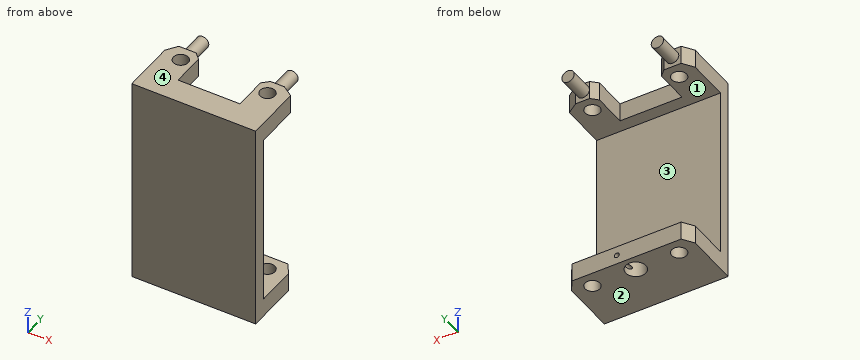
from build123d import *
from OCP.BRepFilletAPI import BRepFilletAPI_MakeChamfer

# Parameters (mm, degrees)
SKETCH1_W                      = 100
SKETCH1_H                      = 52
BOSS_EXTRUDE1_DEPTH            = 15
SKETCH2_R                      = 6
BOSS_EXTRUDE2_DEPTH            = 140
SKETCH3_W                      = 100
SKETCH3_H                      = 46
BOSS_EXTRUDE3_DEPTH            = 15
SKETCH4_W                      = 100
SKETCH4_H                      = 15
BOSS_EXTRUDE4_DEPTH            = 6
SKETCH5_W                      = 100
SKETCH5_H                      = 10
BOSS_EXTRUDE5_DEPTH            = 30
SKETCH6_W                      = 100
SKETCH6_H                      = 10
BOSS_EXTRUDE6_DEPTH            = 30
SKETCH7_W                      = 50
SKETCH7_H                      = 32
CUT_EXTRUDE1_DEPTH             = 168.705098312
SKETCH8_W                      = 6
SKETCH8_H                      = 1
SKETCH9_W                      = 6
SKETCH9_H                      = 1
SKETCH10_W                     = 6
SKETCH10_H                     = 1
SKETCH11_W                     = 6
SKETCH11_H                     = 1
SKETCH12_W                     = 6
SKETCH12_H                     = 140
F_10_0_10_DIAMETER_HOLE1_D     = 10
F_10_0_10_DIAMETER_HOLE1_DEPTH = 10
F_4_0_4_DIAMETER_HOLE1_D       = 4
F_4_0_4_DIAMETER_HOLE1_DEPTH   = 20
F_16_0_16_DIAMETER_HOLE1_D     = 16
F_16_0_16_DIAMETER_HOLE1_DEPTH = 16
CHAMFER1_SIZE                  = 8.75
CHAMFER1_SIZE2                 = 6
CHAMFER2_SIZE                  = 5
SKETCH19_R                     = 6
CUT_EXTRUDE2_DEPTH             = 300
SKETCH20_W                     = 80
SKETCH20_H                     = 10
BOSS_EXTRUDE7_DEPTH            = 100
SKETCH21_R                     = 5
BOSS_EXTRUDE8_DEPTH            = 10
SKETCH23_R                     = 5
BOSS_EXTRUDE10_DEPTH           = 20
SKETCH24_R                     = 8.075
CUT_EXTRUDE3_DEPTH             = 40
SKETCH25_R                     = 6.025
CUT_EXTRUDE4_DEPTH             = 187


with BuildPart() as part:
    # Sketch1 → Boss-Extrude1 (new body)
    with BuildSketch(Plane.XY.offset(85)):
        with Locations((0, -14)):
            Rectangle(SKETCH1_W, SKETCH1_H)
    extrude(amount=-BOSS_EXTRUDE1_DEPTH)

    # Sketch2 → Boss-Extrude2 (add)
    with BuildSketch(Plane(origin=(0, 0, 70), x_dir=(-1, 0, 0), z_dir=(0, 0, -1))):
        with Locations(Location((35, 0, 0), (0, 0, 180))):
            Circle(SKETCH2_R)
    extrude(amount=BOSS_EXTRUDE2_DEPTH)

    # Sketch3 → Boss-Extrude3 (add)
    with BuildSketch(Plane.XY.offset(-70)):
        with Locations((0, -17)):
            Rectangle(SKETCH3_W, SKETCH3_H)
    extrude(amount=-BOSS_EXTRUDE3_DEPTH)

    # Sketch4 → Boss-Extrude4 (add)
    with BuildSketch(Plane(origin=(0, 6, 0), x_dir=(-1, 0, 0), z_dir=(0, 1, 0))):
        with Locations((0, -77.5)):
            Rectangle(SKETCH4_W, SKETCH4_H)
    extrude(amount=BOSS_EXTRUDE4_DEPTH)

    # Sketch5 → Boss-Extrude5 (add)
    with BuildSketch(Plane(origin=(0, 0, 70), x_dir=(-1, 0, 0), z_dir=(0, 0, -1))):
        with Locations((0, -35)):
            Rectangle(SKETCH5_W, SKETCH5_H)
    extrude(amount=BOSS_EXTRUDE5_DEPTH)

    # Sketch6 → Boss-Extrude6 (add)
    with BuildSketch(Plane.XY.offset(-70)):
        with Locations((0, -35)):
            Rectangle(SKETCH6_W, SKETCH6_H)
    extrude(amount=BOSS_EXTRUDE6_DEPTH)

    # Sketch7 → Cut-Extrude1 (cut, through all)
    with BuildSketch(Plane(origin=(0, 0, 70), x_dir=(-1, 0, 0), z_dir=(0, 0, -1))):
        with Locations((0, -4)):
            Rectangle(SKETCH7_W, SKETCH7_H)
    extrude(amount=-CUT_EXTRUDE1_DEPTH, mode=Mode.SUBTRACT)

    # Sketch8 → Revolve1 (revolve)
    with BuildSketch(Plane(origin=(0, 0, 0), x_dir=(1, 0, 0), z_dir=(0, 1, 0))):
        with Locations((38, 85.5)):
            Rectangle(SKETCH8_W, SKETCH8_H)
    revolve(axis=Axis((35, 0, -86), (0, 0, 1)))

    # Sketch9 → Revolve2 (revolve)
    with BuildSketch(Plane(origin=(0, 0, 0), x_dir=(1, 0, 0), z_dir=(0, 1, 0))):
        with Locations((-32, 85.5)):
            Rectangle(SKETCH9_W, SKETCH9_H)
    revolve(axis=Axis((-35, 0, -86), (0, 0, 1)))

    # Sketch10 → Revolve3 (revolve)
    with BuildSketch(Plane(origin=(0, 0, 0), x_dir=(1, 0, 0), z_dir=(0, 1, 0))):
        with Locations((38, -85.5)):
            Rectangle(SKETCH10_W, SKETCH10_H)
    revolve(axis=Axis((35, 0, 85), (0, 0, 1)))

    # Sketch11 → Revolve4 (revolve)
    with BuildSketch(Plane(origin=(0, 0, 0), x_dir=(1, 0, 0), z_dir=(0, 1, 0))):
        with Locations((-32, -85.5)):
            Rectangle(SKETCH11_W, SKETCH11_H)
    revolve(axis=Axis((-35, 0, 85), (0, 0, 1)))

    # Sketch12 → Revolve5 (revolve)
    with BuildSketch(Plane(origin=(0, 0, 0), x_dir=(1, 0, 0), z_dir=(0, 1, 0))):
        with Locations((38, 0)):
            Rectangle(SKETCH12_W, SKETCH12_H)
    revolve(axis=Axis((35, 0, -70), (0, 0, 1)))

    # Ø10.0 (10) Diameter Hole1
    with Locations(Plane(origin=(0, -40, 0), x_dir=(-1, 0, 0), z_dir=(0, -1, 0))):
        with Locations((35, -55), (-35, -55), (-35, 54.99817447), (35, 54.99817447)):
            Hole(F_10_0_10_DIAMETER_HOLE1_D / 2, depth=F_10_0_10_DIAMETER_HOLE1_DEPTH)

    # Ø4.0 (4) Diameter Hole1
    with Locations(Plane(origin=(0, 12, 0), x_dir=(1, 0, 0), z_dir=(0, 1, 0))):
        with Locations((8, 77.5)):
            Hole(F_4_0_4_DIAMETER_HOLE1_D / 2, depth=F_4_0_4_DIAMETER_HOLE1_DEPTH)

    # Ø16.0 (16) Diameter Hole1
    with Locations(Plane.XY.offset(-70)):
        with Locations((0, 0)):
            Hole(F_16_0_16_DIAMETER_HOLE1_D / 2, depth=F_16_0_16_DIAMETER_HOLE1_DEPTH)

    # Chamfer1: one chamfer whose edges measure the first distance from different faces: ONE call of the kernel's chamfer builder (chamfer() names one face for all edges)
    chamfer1_edges_1 = [part.edges().sort_by_distance(p)[0] for p in [
        (50, 12, -77.5),
    ]]
    chamfer1_side_1 = [part.faces().sort_by_distance(p)[0] for p in [
        (50, -19.833333333, -71.25),
    ]]
    chamfer1_edges_2 = [part.edges().sort_by_distance(p)[0] for p in [
        (-50, 12, -77.5),
    ]]
    chamfer1_side_2 = [part.faces().sort_by_distance(p)[0] for p in [
        (-50, -19.833333333, -71.25),
    ]]
    chamfer1_edges_3 = [part.edges().sort_by_distance(p)[0] for p in [
        (-50, 12, 77.5),
    ]]
    chamfer1_side_3 = [part.faces().sort_by_distance(p)[0] for p in [
        (-50, -19.833333333, 71.25),
    ]]
    chamfer1_edges_4 = [part.edges().sort_by_distance(p)[0] for p in [
        (50, 12, 77.5),
    ]]
    chamfer1_side_4 = [part.faces().sort_by_distance(p)[0] for p in [
        (37.5, 12, 77.5),
    ]]
    chamfer1 = BRepFilletAPI_MakeChamfer(part.part.solid().wrapped)
    for e in chamfer1_edges_1:
        chamfer1.Add(CHAMFER1_SIZE, CHAMFER1_SIZE2, e.wrapped, chamfer1_side_1[0].wrapped)  # the first distance lies on this face
    for e in chamfer1_edges_2:
        chamfer1.Add(CHAMFER1_SIZE, CHAMFER1_SIZE2, e.wrapped, chamfer1_side_2[0].wrapped)  # the first distance lies on this face
    for e in chamfer1_edges_3:
        chamfer1.Add(CHAMFER1_SIZE, CHAMFER1_SIZE2, e.wrapped, chamfer1_side_3[0].wrapped)  # the first distance lies on this face
    for e in chamfer1_edges_4:
        chamfer1.Add(CHAMFER1_SIZE, CHAMFER1_SIZE2, e.wrapped, chamfer1_side_4[0].wrapped)  # the first distance lies on this face
    add(Compound.cast(chamfer1.Shape()), mode=Mode.REPLACE)

    # Chamfer2
    chamfer2_edges = [part.edges().sort_by_distance(p)[0] for p in [
        (-25, 12, 77.5),
        (25, 12, 77.5),
    ]]
    chamfer(chamfer2_edges, length=CHAMFER2_SIZE)

    # Sketch19 → Cut-Extrude2 (cut)
    with BuildSketch(Plane(origin=(0, 0, -86), x_dir=(-1, 0, 0), z_dir=(0, 0, -1))):
        with Locations(Location((-35, 0, 0), (0, 0, 180))):
            Circle(SKETCH19_R)
        with Locations(Location((35, 0, 0), (0, 0, 180))):
            Circle(SKETCH19_R)
    extrude(amount=-CUT_EXTRUDE2_DEPTH, mode=Mode.SUBTRACT)


with BuildPart() as cut_extrude2_piece_1:
    # of the separate pieces the step leaves, piece 1, a body of its own (cut_extrude2_pieces)
    add(part.part.solids().sort_by_distance((-50, 3.25, -70))[0])



with BuildPart() as cut_extrude2_piece_2:
    # of the separate pieces the step leaves, piece 2, a body of its own (cut_extrude2_pieces)
    add(part.part.solids().sort_by_distance((30, 12, 70))[0])


with BuildPart() as cut_extrude2_piece_1_1:
    add(cut_extrude2_piece_1.part)

    add(cut_extrude2_piece_2.part)  # Boss-Extrude7 merges Cut-Extrude2 piece 2
    # Sketch20 → Boss-Extrude7 (add)
    with BuildSketch(Plane.ZY.offset(50)):
        with Locations((0, -35)):
            Rectangle(SKETCH20_W, SKETCH20_H)
    extrude(amount=-BOSS_EXTRUDE7_DEPTH)

    # Sketch21 → Boss-Extrude8 (add)
    with BuildSketch(Plane(origin=(0, -30, 0), x_dir=(1, 0, 0), z_dir=(0, 1, 0))):
        with Locations((-35, 54.99817447)):
            Circle(SKETCH21_R)
        with Locations((35, 54.99817447)):
            Circle(SKETCH21_R)
        with Locations((35, -55)):
            Circle(SKETCH21_R)
        with Locations((-35, -55)):
            Circle(SKETCH21_R)
    extrude(amount=-BOSS_EXTRUDE8_DEPTH)

    # Sketch23 → Boss-Extrude10 (add)
    with BuildSketch(Plane(origin=(0, 12, 0), x_dir=(1, 0, 0), z_dir=(0, 1, 0))):
        with Locations(Location((-37.07435596, -77.890606879, 0), (0, 0, 270))):
            Circle(SKETCH23_R)
        with Locations(Location((35.083214943, -77.890606879, 0), (0, 0, 270))):
            Circle(SKETCH23_R)
    extrude(amount=BOSS_EXTRUDE10_DEPTH)

    # Sketch24 → Cut-Extrude3 (cut)
    with BuildSketch(Plane(origin=(0, 0, -85), x_dir=(-1, 0, 0), z_dir=(0, 0, -1))):
        Circle(SKETCH24_R)
    extrude(amount=-CUT_EXTRUDE3_DEPTH, mode=Mode.SUBTRACT)

    # Sketch25 → Cut-Extrude4 (cut)
    with BuildSketch(Plane.XY.offset(85)):
        with Locations((-35, 0)):
            Circle(SKETCH25_R)
        with Locations((35, 0)):
            Circle(SKETCH25_R)
    extrude(amount=-CUT_EXTRUDE4_DEPTH, mode=Mode.SUBTRACT)


solid = cut_extrude2_piece_1_1.part
The model under review builds one solid part; all positions refer to its coordinate system, in mm. Face numbers are marked on the shaded views. Give positions to 0.01 mm unless a question says otherwise; leave off trailing zeros. Loops run counter-clockwise (first coordinate to the right, second up) from the corner with the lowest first, then second, coordinate; pieces in that order, holes last. Notation, with made-up numbers: (70, 5) -> (78, 5) arc R19 ccw to (78, 26) -> close; hole circle Ø4 at (-4, 62.5). An arc over 180 degrees is marked (long way). Put each result on its own line as item: value. Start each with the question number.
1. Mouldability with a two-part tool opening along Z and no side actions: class the marked faces 1, 2, 3 and 4 as released by +Z, released by -Z, zero draft, split by the parting line, or undercut.
2. Clearance check with flat-ended pins moving along their axes: P1, Ø3, axis at x = 8, z = -77.5, coming from the +Y side; P2, Ø11, axis at x = -35, y = 0, coming from the -Z side; P3, Ø15.5, axis at x = -35, y = 0, coming from the -Z side; P4, Ø10, axis at x = 39.5, z = 28.5, coming from the +Y side. State where each tip first meets the part, or that it passes through.
3. We need section C-C on z = -77.5. State the section outline as (x, y) points (3 decimals), then the cut area to 3 significant figures.
4. We need section A-A on y = -23. State the section outline as (x, z) points.
5. We need section D-D on y = 0. State how many separate pieces and enclosed holes the cut face has, then the cut area to 3 significant figures.
6. Wall thickness on probe 1 along Z at (x, y) = (-41, 6.5); probe 2 along Y at (x, z) = (0, -73.25) (3 decimals); probe 3 along Y at (x, z) = (-35, 75.25) (3 decimals): over which ranges is each line inside the solid? List them lowest first.
7. We need section B-B on x = 0. State the section outline as (y, z) points (3 decimals).
Determined:
1. face 1: undercut
1. face 2: released by -Z
1. face 3: undercut
1. face 4: released by +Z
2. P1: y = -8
2. P2: through
2. P3: z = -85
2. P4: y = -30
3. outline: (-50, -40) -> (50, -40) -> (50, 3.25) -> (44, 12) -> (10, 12) -> (10, -8) -> (6, -8) -> (6, -5.404) arc R8.075 cw (long way) to (6, 5.404) -> (6, 12) -> (-44, 12) -> (-50, 3.25) -> close; hole circle Ø12.05 at (-35, 0); hole circle Ø12.05 at (35, 0)
3. area: 4,650 mm^2
4. outline: (-50, -85) -> (50, -85) -> (50, -70) -> (-50, -70) -> close; (-50, 70) -> (50, 70) -> (50, 85) -> (-50, 85) -> close
5. separate pieces: 8
5. enclosed holes: 0
5. area: 1,280 mm^2
6. probe 1: -85 to -70, 70 to 85
6. probe 2: -40 to -8.075, 8.075 to 12
6. probe 3: -40 to -6.025, 6.025 to 32
7. outline: (-40, -85) -> (-8.075, -85) -> (-8.075, -70) -> (-30, -70) -> (-30, 70) -> (-20, 70) -> (-20, 85) -> (-40, 85) -> close; (8.075, -85) -> (12, -85) -> (12, -70) -> (8.075, -70) -> close
